```python
from build123d import *

# Parameters (mm, degrees)
SKETCH1_R           = 75
BOSS_EXTRUDE1_DEPTH = 25
SKETCH2_R           = 8
BOSS_EXTRUDE2_DEPTH = 35
SKETCH3_R           = 10
BOSS_EXTRUDE3_DEPTH = 10
CHAMFER1_SIZE       = 5
SKETCH4_R           = 53
SKETCH4_R_2         = 8
CUT_EXTRUDE1_DEPTH  = 1


with BuildPart() as part:
    # Sketch1 → Boss-Extrude1 (new body, symmetric)
    with BuildSketch(Plane(origin=(0, 0, 0), x_dir=(0, 0, -1), z_dir=(1, 0, 0))):
        Circle(SKETCH1_R)
    extrude(amount=BOSS_EXTRUDE1_DEPTH, both=True)

    # Sketch2 → Boss-Extrude2 (add, symmetric)
    with BuildSketch(Plane(origin=(0, 0, 0), x_dir=(0, 0, -1), z_dir=(1, 0, 0))):
        Circle(SKETCH2_R)
    extrude(amount=BOSS_EXTRUDE2_DEPTH, both=True)

    # Sketch3 → Boss-Extrude3 (add)
    with BuildSketch(Plane(origin=(35, 0, 0), x_dir=(0, 0, -1), z_dir=(1, 0, 0))):
        Circle(SKETCH3_R)
    boss_extrude3 = extrude(amount=BOSS_EXTRUDE3_DEPTH)

    # Mirror1: Boss-Extrude3 across plane
    add(boss_extrude3.mirror(Plane(origin=(0, 0, 0), x_dir=(0, 0, 1), z_dir=(1, 0, 0))))

    # Chamfer1
    chamfer1_edges = [part.edges().sort_by_distance(p)[0] for p in [
        (-25, 0, 75),
        (25, 0, 75),
    ]]
    chamfer(chamfer1_edges, length=CHAMFER1_SIZE)

    # Sketch4 → Cut-Extrude1 (cut)
    with BuildSketch(Plane(origin=(25, 0, 0), x_dir=(0, 0, -1), z_dir=(1, 0, 0))):
        Circle(SKETCH4_R)
        Circle(SKETCH4_R_2, mode=Mode.SUBTRACT)
    cut_extrude1 = extrude(amount=-CUT_EXTRUDE1_DEPTH, mode=Mode.SUBTRACT)

    # Mirror2: Cut-Extrude1 across plane
    add(cut_extrude1.mirror(Plane(origin=(0, 0, 0), x_dir=(0, 0, 1), z_dir=(1, 0, 0))), mode=Mode.SUBTRACT)

    # Sketch5 → Revolve1 (revolve)
    with BuildSketch(Plane(origin=(0, 0, 0), x_dir=(1, 0, 0), z_dir=(0, 1, 0))):
        with BuildLine():
            Line((24, 0), (24, 50.661166178))
            add(Edge.make_bspline(
                [(27, 0), (28.099596194, 25.463923128), (24, 50.661166178)],
                knots=[0, 0, 0, 1, 1, 1], degree=2))
            Line((27, 0), (24, 0))
        make_face()
    revolve1 = revolve(axis=Axis((27, 0, 0), (1, 0, 0)))

    # Mirror3: Revolve1 across plane
    add(revolve1.mirror(Plane(origin=(0, 0, 0), x_dir=(0, 0, 1), z_dir=(1, 0, 0))))


solid = part.part
```
Part model, mm, in its own coordinate system. A direction names the side the tool comes from. Give positions to 0.01 mm unless a question says otherwise; leave off trailing zeros. Loops run counter-clockwise (first coordinate to the right, second up) from the corner with the lowest first, then second, coordinate; pieces in that order, holes last. Notation, with made-up numbers: M 69,-38 L 121,-38 A6 cw 121,-34 Z; hole C 87.5,43.5 d7. An arc over 180 degrees is marked long. Return JSON: item names as keys, results as strings.
1) Drill centre lines: line 1 (X direction, y = -12, z = -51.5); line 2 (X direction, y = -49.5, z = -39); line 3 (Z direction, x = 0.5, y = 60.5). Where is each one in solid material? Low to high.
Calculated:
{"line 1": "x = -24 to 24", "line 2": "x = -25 to 25", "line 3": "z = -44.33 to 44.33"}
2) 3-axis set-ups, long thin cutter, end or side, ignore diameter. For faces 5 (the face through (-39.93, -9.76, 2.17)), 6 (the face through (39.93, -9.76, 2.17)), 7 (the face through (-31.05, -7.81, 1.73)): which of +Z, -Z, +X, -X, +Y, -Y reach the whole face in a straight line?
Calculated:
{"face 5": "-X", "face 6": "+X", "face 7": "none"}
3) Pull direction X, two halves, no side cores. Call faces 1 (the face through (-24.51, 44.69, -28.49)), 2 (the face through (31.16, -7.81, 1.73)), 3 (the face through (45, 0, 0)), 4 (the face through (-25, 52, 11)): released by +X, released by -X, zero draft, split by the parting line, or undercut.
Calculated:
{"face 1": "zero draft", "face 2": "undercut", "face 3": "released by +X", "face 4": "released by -X"}
4) Saw through at A-A, the plane x = -6. List the corners of the cut face in (y, z).
Calculated:
{"outline": "C 0,0 d150"}
5) Flat gauge pins, fed straight in: pin 1 Ø2 at (y, z) = (-59.5, 22) entering from -X; pin 2 Ø1.5 at (x, y) = (13, 17) entering from +Z; pin 3 Ø1.5 at (y, z) = (2.5, -52.5) entering from +X. Where does each tip first touch, or does it go through?
Calculated:
{"pin 1": "stops at x = -25", "pin 2": "stops at z = 73.22", "pin 3": "stops at x = 25"}
